from build123d import *

# Parameters (mm, degrees)
BASE_FLANGE2_DEPTH           = 1.5
EDGE_FLANGE1_STRIP_W         = 10
EDGE_FLANGE1_STRIP_H         = 1.5
EDGE_FLANGE1_STRIP_CUT_DEPTH = 330
EDGE_FLANGE1_DEPTH           = 330
CUT_EXTRUDE1_DEPTH           = 174.399106111
CUT_EXTRUDE1_DEPTH_BACK      = 10


# Sheet-metal steps are written as plain solids
with BuildPart() as part:
    # Sketch1 → Base-Flange2 (new body)
    with BuildSketch(Plane.XY):
        Polygon((-165, 10), (165, 10), (165, -5), (50, -50), (-50, -50), (-165, -5), align=None)
    extrude(amount=-BASE_FLANGE2_DEPTH)

    # Edge-Flange1 strip (across the edge) → Edge-Flange1 strip cut (cut)
    with BuildSketch(Plane(origin=(165, 10, 0), x_dir=(0, -1, 0), z_dir=(-1, 0, 0))):
        with Locations((-1.5, -0.75)):
            Rectangle(EDGE_FLANGE1_STRIP_W, EDGE_FLANGE1_STRIP_H)
    extrude(amount=EDGE_FLANGE1_STRIP_CUT_DEPTH, mode=Mode.SUBTRACT)

    # Edge-Flange1 section (across the edge) → Edge-Flange1 (add)
    with BuildSketch(Plane(origin=(165, 10, 0), x_dir=(0, -1, 0), z_dir=(-1, 0, 0))):
        with BuildLine():
            Line((0, 2), (0, 18.5))
            Line((0, 18.5), (1.5, 18.5))
            Line((1.5, 18.5), (1.5, 2))
            ThreePointArc((1.5, 2), (2.085786438, 0.585786438), (3.5, 0))
            Line((3.5, 0), (3.5, -1.5))
            ThreePointArc((3.5, -1.5), (1.025126266, -0.474873734), (0, 2))
        make_face()
    extrude(amount=EDGE_FLANGE1_DEPTH)

    # Sketch13 → Cut-Extrude1 (cut, two sides: drawn at the far end of the back side and taken through both)
    with BuildSketch(Plane.XY.offset(-CUT_EXTRUDE1_DEPTH_BACK)):
        with BuildLine():
            Line((-13.5, -3.5), (-13.5, 21.0126417))
            Line((-13.5, 21.0126417), (13.5, 21.0126417))
            Line((13.5, 21.0126417), (13.5, -3.5))
            ThreePointArc((13.5, -3.5), (0, -17), (-13.5, -3.5))
        make_face()
    extrude(amount=CUT_EXTRUDE1_DEPTH + CUT_EXTRUDE1_DEPTH_BACK, mode=Mode.SUBTRACT)


solid = part.part
CAD build for the part. Positions are in the model's coordinates, mm. A direction names the side the tool comes from. Round coordinates to 2 decimals unless told otherwise and drop trailing zeros. Loops run counter-clockwise (first coordinate to the right, second up) from the corner with the lowest first, then second, coordinate; pieces in that order, holes last.
(1) Two-plate mould, pull along X, no slides. Class faces 4 (the flat face through (2, -21, -1.5)), 5 (the flat face through (108.305, -27.185, -0.74)), 6 (the flat face through (-13.5, 9, 5)): +X half, -X half, draft (parallel to the pull), parting line (faces both ways), or undercut.
(2) Drop flat-ended pins along their axis: pin 1 (11 mm diameter, centred on y = 0.5, z = 4.5, fed in from +X); pin 2 (17 mm diameter, centred on x = -6, y = -15.5, fed in from +Z); pin 3 (5 mm diameter, centred on x = 86, z = 7, fed in from -Y). Give the stop position or say it passes through.
(3) Cut at B-B (x = -138). Give the cut face in (y, z).
(4) Which spindle directions (+Z, -Z, +X, -X, +Y, -Y) get a long thin tool onto all of the face, cutting with end or side? Do faces 1 (the flat face through (-165, 9, 5)), 2 (the flat face through (13.5, 9, 5)), 3 (the flat face through (90, 8.5, 10)). Say none if no direction does.
(5) Cut at C-C (y = -39.5). Give the cut face in (x, z), plus the area to 4 significant figures.
(6) Wall check: line 1 along Y through (x, z) = (118, 13.5); line 2 along Z through (x, y) = (81, -26.5); line 3 along Y through (x, z) = (-48, 0.75). Give the ranges that are in metal, low to high.
(7) Cut at A-A (z = 7.25). Give the cut face in (x, y).
(8) Cut at D-D (x = 0). Give the cut face in (y, z), plus the area to 3 significant figures.
Findings below:
1. face 4: draft
1. face 5: +X half
1. face 6: undercut
2. pin 1: stops at x = 165
2. pin 2: stops at z = 0
2. pin 3: stops at y = 8.5
3. outline: (-15.57, -1.5) - (6.5, -1.5) arc R3.5 ccw to (10, 2) - (10, 18.5) - (8.5, 18.5) - (8.5, 2) arc R2 cw to (6.5, 0) - (-15.57, 0) - close
4. face 1: +Z, -Z, -X, +Y, -Y
4. face 2: +Z, -Z, +Y
4. face 3: +Z, +X, -X, -Y
5. outline: (-76.83, -1.5) - (76.83, -1.5) - (76.83, 0) - (-76.83, 0) - close
5. area: 230.5 mm2
6. line 1: y = 8.5 to 10
6. line 2: z = -1.5 to 0
6. line 3: y = 8.06 to 9.77
7. outline: (-165, 8.5) - (-13.5, 8.5) - (-13.5, 10) - (-165, 10) - close; (13.5, 8.5) - (165, 8.5) - (165, 10) - (13.5, 10) - close
8. outline: (-50, -1.5) - (-17, -1.5) - (-17, 0) - (-50, 0) - close
8. area: 49.5 mm2
